from build123d import *

# Parameters (mm, degrees)
EXTRUDE_1_DEPTH     = 6
CUT_EXTRUDE_3_REACH = 8
SKETCH_2_R          = 2
SKETCH_2_W          = 8
SKETCH_2_H          = 2
CHAMFER_1_SIZE      = 3
SKETCH_5_W          = 9
SKETCH_5_H          = 6
EXTRUDE_5_DEPTH     = 25
CHAMFER_3_SIZE      = 12
CHAMFER_3_SIZE2     = 5.595691898


with BuildPart() as part:
    # 草图1 → 凸台-拉伸1 (new body)
    with BuildSketch(Plane(origin=(0, 0, 0), x_dir=(1, 0, 0), z_dir=(0, 1, 0))):
        Polygon((-4, 5), (-4, 10), (-10, 10), (-10, 5), (-10, 0), (10, 0), (10, 5), (10, 10), (4, 10), (4, 5), align=None)
    extrude(amount=EXTRUDE_1_DEPTH)

    # 草图2 → 切除-拉伸3 (cut, up to next)
    with BuildSketch(Plane(origin=(0, 6, 0), x_dir=(1, 0, 0), z_dir=(0, 1, 0)), mode=Mode.PRIVATE) as cut_extrude_3_sk1:
        with Locations((-7, 7)):
            Circle(SKETCH_2_R)
    cut_extrude_3_tool1 = extrude(cut_extrude_3_sk1.sketch, amount=-CUT_EXTRUDE_3_REACH, mode=Mode.PRIVATE) & part.part
    add(cut_extrude_3_tool1.solids().sort_by_distance((-7, 6, -7))[0], mode=Mode.SUBTRACT)
    # 草图2 → 切除-拉伸3 (cut, up to next)
    with BuildSketch(Plane(origin=(0, 6, 0), x_dir=(1, 0, 0), z_dir=(0, 1, 0)), mode=Mode.PRIVATE) as cut_extrude_3_sk2:
        with Locations((7, 7)):
            Circle(SKETCH_2_R)
    cut_extrude_3_tool2 = extrude(cut_extrude_3_sk2.sketch, amount=-CUT_EXTRUDE_3_REACH, mode=Mode.PRIVATE) & part.part
    add(cut_extrude_3_tool2.solids().sort_by_distance((7, 6, -7))[0], mode=Mode.SUBTRACT)
    # 草图2 → 切除-拉伸3 (cut, up to next)
    with BuildSketch(Plane(origin=(0, 6, 0), x_dir=(1, 0, 0), z_dir=(0, 1, 0)), mode=Mode.PRIVATE) as cut_extrude_3_sk3:
        with Locations((0, 2)):
            Rectangle(SKETCH_2_W, SKETCH_2_H)
    cut_extrude_3_tool3 = extrude(cut_extrude_3_sk3.sketch, amount=-CUT_EXTRUDE_3_REACH, mode=Mode.PRIVATE) & part.part
    add(cut_extrude_3_tool3.solids().sort_by_distance((0, 6, -2))[0], mode=Mode.SUBTRACT)

    # 倒角1
    chamfer_1_edges = [part.edges().sort_by_distance(p)[0] for p in [
        (10, 3, 0),
        (-10, 3, 0),
    ]]
    chamfer(chamfer_1_edges, length=CHAMFER_1_SIZE)

    # 草图5 → 凸台-拉伸5 (add)
    with BuildSketch(Plane.XZ):
        with Locations((0, -7)):
            Rectangle(SKETCH_5_W, SKETCH_5_H)
    extrude(amount=EXTRUDE_5_DEPTH)

    # 倒角3
    chamfer_3_edges = [part.edges().sort_by_distance(p)[0] for p in [
        (4.5, -25, -7),
    ]]
    chamfer_3_side = [part.faces().sort_by_distance(p)[0] for p in [
        (4.5, -12.5, -7),
    ]]
    chamfer(chamfer_3_edges, length=CHAMFER_3_SIZE, length2=CHAMFER_3_SIZE2, reference=chamfer_3_side[0])


solid = part.part
Input: part model. Units: mm. Frame: model coordinates. A direction names the side the tool comes from. Give positions to 0.01 mm unless a question says otherwise; leave off trailing zeros. Loops run counter-clockwise (first coordinate to the right, second up) from the corner with the lowest first, then second, coordinate; pieces in that order, holes last. Notation, with made-up numbers: (86.5, -10.75) - (95.5, -10.75) arc R16 cw to (95.5, 16.25) - close; hole circle Ø10 at (45.5, 52.25). An arc over 180 degrees is marked (long way). Use CSV: the item, a comma, the result in double quotes. Start each with the question number.
Item 1: Section C-C on x = -7.5. Return loops of the section in (y, z), then the cut area to 3 significant figures.
Item 2: Contact query for flat-ended pins moving along their axis: P1, Ø5, axis at y = -8.5, z = -6.5, coming from the +X side; P2, Ø5, axis at x = 1, y = 3.5, coming from the -Z side; P3, Ø4.5, axis at x = -0.5, y = -12, coming from the +Z side; P4, Ø3.5, axis at x = 7, z = -7, coming from the -Y side. Output: stop coordinate, or through.
Item 3: Line query: line 1 (X direction, y = 1.9, z = -7); line 2 (Z direction, x = 7, y = 4.7); line 3 (Y direction, x = -6.5, z = -9.5). Output: solid intervals per line, ascending.
Item 4: Section D-D on y = -4. Return loops of the section in (x, z).
Item 5: Mould query, pull axis X, two halves, no side actions, for faces 1 (the flat face through (-3, -25, -7)), 2 (the flat face through (-8, 3, -1)), 3 (the flat face through (4.5, -6, -7)), 4 (the cylindrical face through (-9, 3, -7)). Classes: pulls with the +X half, pulls with the -X half, needs draft (parallel to the pull), parting line crosses it, or undercut.
Item 6: Reachability of faces 5 (the flat face through (0, 3, -3)), 6 (the flat face through (10, 3, -6)), 7 (the flat face through (-4.5, -12, -7)), 8 (the flat face through (0, 3, 0)), 9 (the flat face through (0, 0, -7)) from +Z, -Z, +X, -X, +Y, -Y: full face, straight path, thin tool, end or side. Return the list, or none.
Item 7: Section A-A on z = -7. Return loops of the section in (x, y).
Item 8: Section B-B on y = 2. Return loops of the section in (x, z), then the cut area to 3 significant figures.
Ans:
1,outline,"(0, -10) - (6, -10) - (6, -8.94) - (0, -8.94) - close; (0, -5.06) - (6, -5.06) - (6, -0.5) - (0, -0.5) - close"
1,area,"33.8 mm2"
2,P1,"stops at x = 4.5"
2,P2,"stops at z = -5"
2,P3,"stops at z = -4"
2,P4,"passes through"
3,line 1,"x = -10 to -9, -5 to -4, 4 to 5, 9 to 10"
3,line 2,"z = -10 to -9, -5 to 0"
3,line 3,"y = 0 to 6"
4,outline,"(-4.5, -10) - (4.5, -10) - (4.5, -4) - (-4.5, -4) - close"
5,face 1,"needs draft"
5,face 2,"pulls with the -X half"
5,face 3,"pulls with the +X half"
5,face 4,"undercut"
6,face 5,"+Y, -Y"
6,face 6,"+Z, -Z, +X, +Y, -Y"
6,face 7,"+Z, -Z, -X, -Y"
6,face 8,"+Z, +X, -X, +Y, -Y"
6,face 9,"-Z, +Y"
7,outline,"(-10, 0) - (-9, 0) - (-9, 6) - (-10, 6) - close; (-5, 0) - (-4.5, 0) - (-4.5, -25) - (-1.1, -25) - (4.5, -13) - (4.5, 0) - (5, 0) - (5, 6) - (4, 6) - (4, 0) - (-4, 0) - (-4, 6) - (-5, 6) - close; (9, 0) - (10, 0) - (10, 6) - (9, 6) - close"
8,outline,"(-10, -10) - (-4, -10) - (-4, -5) - (4, -5) - (4, -10) - (10, -10) - (10, -3) - (7, 0) - (-7, 0) - (-10, -3) - close; hole circle Ø4 at (-7, -7); hole (-4, -3) - (4, -3) - (4, -1) - (-4, -1) - close; hole circle Ø4 at (7, -7)"
8,area,"110 mm2"
